Design review of the part built by this model. Coordinates are the model's own, in mm. Face numbers are marked on the shaded views. A direction names the side the tool comes from. Coordinates: 2 decimals unless noted, no trailing zeros. Write each loop counter-clockwise with the first axis right and the second up, starting at its lowest first coordinate (ties: lowest second). Pieces come first, ordered by that corner, then holes. Notation, with made-up numbers: (11, -31.75) - (41, -31.75) arc R5 cw to (41, -23.75) - close; hole circle Ø2 at (-9, -14). An arc over 180 degrees is marked (long way). Answer as a JSON object with one key per item and string values.
Autodesk Inventor part; units mm, degrees
ref_plane "YZ Plane" through (0, 0, 0) normal (1, 0, 0) x (0, 1, 0)
ref_plane "XZ Plane" through (0, 0, 0) normal (0, 1, 0) x (-1, 0, 0)
ref_plane "XY Plane" through (0, 0, 0) normal (0, 0, 1) x (1, 0, 0)
sketch "Sketch1" plane through (0, 0, 0) normal (0, 1, 0) x (-1, 0, 0)
  line L0 (0, 0) -> (14, 0)
  line L1 (14, 0) -> (14, -14)
  line L2 (14, -14) -> (0, -14)
  line L3 (0, -14) -> (0, 0)
  dimension "d0" = 14
  dimension "d1" = 14
extrude "Extrusion1" add sketch "Sketch1" along normal blind 10
fillet "Fillet2" radius 1 4 edges at (0, 5, 0) (0, 5, -14) (-14, 5, 0) (-14, 5, -14)
shell "Shell1" thickness 1.5 removed faces 1 at (-9.3333, 0, -9)
sketch "Sketch3" plane through (0, 0, 0) normal (0, -1, 0) x (1, 0, 0)
  line L0 (-0.25, -11) -> (-1.25, -11)
  line L1 (-1.25, -11) -> (-1.25, -3)
  line L2 (-1.25, -3) -> (-0.25, -3)
  line L3 (-0.25, -3) -> (-0.25, -11)
  line L4 (0, -1) -> (0, -13)
  line L5 (-13, 0) -> (-1, 0)
  line L6 (-12.75, -11) -> (-13.75, -11)
  line L7 (-13.75, -11) -> (-13.75, -3)
  line L8 (-13.75, -3) -> (-12.75, -3)
  line L9 (-12.75, -3) -> (-12.75, -11)
  line L10 (-14, -13) -> (-14, -1)
  point P0 (0, 0)
  dimension "d13" = 8
  dimension "d14" = 1
  dimension "d15" = 0.25
  dimension "d16" = 3
  dimension "d17" = 1
  dimension "d18" = 8
  dimension "d19" = 0.25
  dimension "d20" = 3
extrude "Extrusion3" add sketch "Sketch3" along normal blind 1.5
sketch "Sketch4" plane through (0, 10, 0) normal (0, 1, 0) x (1, 0, 0)
  line L0 (-10, 10) -> (-4, 10)
  line L1 (-4, 10) -> (-4, 4)
  line L2 (-4, 4) -> (-10, 4)
  line L3 (-10, 4) -> (-10, 10)
  line L4 (-1, 14) -> (-13, 14)
  line L5 (0, 1) -> (0, 13)
  point P0 (0, 0)
  dimension "d23" = 6
  dimension "d24" = 6
  dimension "d25" = 4
  dimension "d26" = 4
extrude "Extrusion4" cut sketch "Sketch4" against normal blind 10
sketch "Sketch5" plane through (-13, 0, 0) normal (0, 0, 1) x (1, 0, 0)
  line L0 (12, 0) -> (0, 0)
  line L1 (2, 0) -> (10, 0)
  line L2 (10, 0) -> (10, 2)
  line L3 (10, 2) -> (2, 2)
  line L4 (2, 2) -> (2, 0)
  line L5 (-1, 10) -> (-1, 0)
  point P0 (13, 0)
  dimension "d29" = 2
  dimension "d30" = 8
  dimension "d31" = 3
extrude "Extrusion5" cut sketch "Sketch5" against normal blind 10
properties part number "Small_Button_Part_Two"
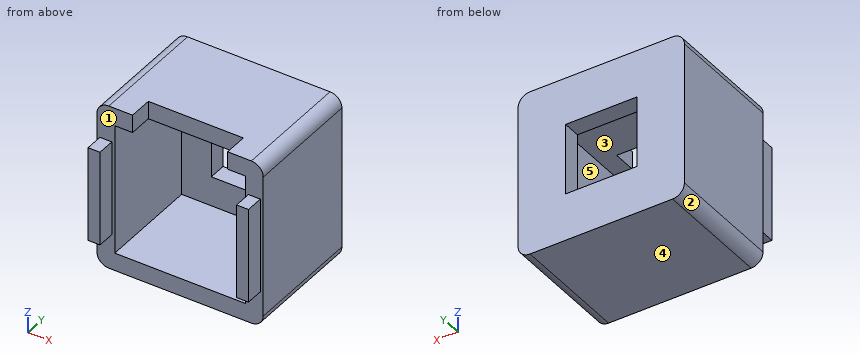
(1) For pin 1 (0.8 mm diameter, centred on x = -0.5, y = -0.5, fed in from -Z); pin 2 (1.2 mm diameter, centred on y = -1, z = -7.5, fed in from +X); pin 3 (1.2 mm diameter, centred on y = -1, z = -7, fed in from -X), all flat-tipped, find the tip position at first contact; note any pin that passes through.
Solved:
{"pin 1": "stops at z = -11", "pin 2": "stops at x = -0.25", "pin 3": "stops at x = -13.75"}
(2) Take a section at B-B, the plane y = 9. Write out the cut boundary in (x, z), and give its area (3 significant figures).
Solved:
{"outline": "(-14, -13) arc R1 ccw to (-13, -14) - (-1, -14) arc R1 ccw to (0, -13) - (0, -1) arc R1 ccw to (-1, 0) - (-13, 0) arc R1 ccw to (-14, -1) - close; hole (-10, -10) - (-4, -10) - (-4, -4) - (-10, -4) - close", "area": "159 mm^2"}
(3) The part is to be moulded in two halves that separate along Z. For the marked faces 1, 2 and 3, say which applies: pulls with the +Z half, pulls with the -Z half, needs draft (parallel to the pull), parting line crosses it, or undercut.
Solved:
{"face 1": "needs draft", "face 2": "pulls with the -Z half", "face 3": "undercut"}
(4) To check wall thickness, follow line 1 (X direction, y = 7.25, z = -9); line 2 (Z direction, x = -5, y = 9.25). State the ranges of each line that lie inside material, in increasing order. Write a range as from..to.
Solved:
{"line 1": "x = -14..-12.5, -1.5..0", "line 2": "z = -14..-10, -4..0"}
(5) Take a section at A-A, the plane z = -5.75. Write out the cut boundary in (x, y).
Solved:
{"outline": "(-14, 0) - (-13.75, 0) - (-13.75, -1.5) - (-12.75, -1.5) - (-12.75, 0) - (-12.5, 0) - (-12.5, 8.5) - (-10, 8.5) - (-10, 10) - (-14, 10) - close; (-4, 8.5) - (-1.5, 8.5) - (-1.5, 0) - (-1.25, 0) - (-1.25, -1.5) - (-0.25, -1.5) - (-0.25, 0) - (0, 0) - (0, 10) - (-4, 10) - close"}
(6) Take a section at D-D, the plane x = -6. Write out the cut boundary in (y, z), and give its area (3 significant figures).
Solved:
{"outline": "(0, -14) - (10, -14) - (10, -10) - (8.5, -10) - (8.5, -12.5) - (0, -12.5) - close; (2, -1.5) - (8.5, -1.5) - (8.5, -4) - (10, -4) - (10, 0) - (2, 0) - close", "area": "34.5 mm^2"}
(7) Take a section at C-C, the plane x = -11.75. Write out the cut boundary in (y, z).
Solved:
{"outline": "(0, -14) - (10, -14) - (10, 0) - (0, 0) - (0, -1.5) - (8.5, -1.5) - (8.5, -12.5) - (0, -12.5) - close"}
(8) Tool access review of the marked faces 4 and 5: name each direction out of +Z, -Z, +X, -X, +Y, -Y from which nothing blocks a thin tool from reaching the whole face with its end or side.
Solved:
{"face 4": "-Z, +X, -X, +Y, -Y", "face 5": "-Y"}
